```python
from build123d import *

# Parameters (mm, degrees)
SKETCH1_W              = 25.4
SKETCH1_H              = 25.4
SKETCH1_W_2            = 19.05
SKETCH1_H_2            = 19.05
EXTRUDE_THIN1_DEPTH    = 101.6
SKETCH2_R              = 9.525
CUT_EXTRUDE1_DEPTH     = 108.763073453
F_10_CLEARANCE_HOLE1_D = 5.1054


with BuildPart() as part:
    # Sketch1 → Extrude-Thin1 (new body)
    with BuildSketch(Plane.XY):
        with Locations((-12.7, 12.7)):
            Rectangle(SKETCH1_W, SKETCH1_H)
        with Locations((-12.7, 12.7)):
            Rectangle(SKETCH1_W_2, SKETCH1_H_2, mode=Mode.SUBTRACT)
    extrude(amount=EXTRUDE_THIN1_DEPTH)

    # Sketch2 → Cut-Extrude1 (cut, through all)
    with BuildSketch(Plane(origin=(0, 0, 0), x_dir=(-1, 0, 0), z_dir=(0, -1, 0))):
        with Locations(Location((12.7, -12.7, 0), (0, 0, 90))):
            Circle(SKETCH2_R)
    extrude(amount=-CUT_EXTRUDE1_DEPTH, mode=Mode.SUBTRACT)

    # #10 Clearance Hole1 (through all)
    with Locations(Plane(origin=(0, 0, 0), x_dir=(0, 0, -1), z_dir=(1, 0, 0))):
        with Locations((-76.2, 12.7), (-88.9, 12.7), (-63.5, 12.7)):
            Hole(F_10_CLEARANCE_HOLE1_D / 2)


solid = part.part
```
Could you check a few things on this model? Use its own coordinates, in mm. A direction names the side the tool comes from. Round coordinates to 2 decimals unless told otherwise and drop trailing zeros. Write each loop counter-clockwise with the first axis right and the second up, starting at its lowest first coordinate (ties: lowest second). Pieces come first, ordered by that corner, then holes. Notation, with made-up numbers: M -8.5,52 L 29.5,52 A21 ccw 29.5,73 Z; hole C -4,48 d3. An arc over 180 degrees is marked long. Write each question's results on one line, items separated by ' | '. Start each with the question number.
1. Imagine slicing it at C-C on z = 63.5. List the corners of the cut face in (x, y) for me (3 decimals).
2. On a 3-axis mill with a long thin cutter (end or side, diameter ignored), from which of +Z, -Z, +X, -X, +Y, -Y can I reach the whole of each face in a straight line? I mean faces 1 (the face through (-3.175, 13, 50)), 2 (the face through (-12.281, 23.79, 22.216)). Say none if no direction works.
3. I need wall thicknesses on L1, parallel to X at y = 21.75, z = 91 (3 decimals); L2, parallel to Y at x = -8, z = 65 (3 decimals); L3, parallel to Y at x = -2, z = 63.5. Which ranges of each line are inside material? Lowest first, please. Write a range as from..to.
4. Imagine slicing it at B-B on y = 7. List the corners of the cut face in (x, z) for me (3 decimals), and give its area (3 significant figures).
5. Imagine slicing it at D-D on y = 12.7. Count the separate pieces of the cut face and the enclosed holes in it, and give its area (3 significant figures).
6. Imagine slicing it at A-A on x = -23.5. List the corners of the cut face in (y, z) for me, and give its area (3 significant figures).
7. Thinking about a two-plate mould opening in X: for faces 3 (the face through (-13, 0, 61)), 4 (the face through (0, 13, 50)), 5 (the face through (-13, 22.225, 57)), which applies, +X half, -X half, draft (parallel to the pull), parting line (faces both ways), or undercut?
Result sheet:
1) outline: M -25.4,0 L 0,0 L 0,10.147 L -3.175,10.147 L -3.175,3.175 L -22.225,3.175 L -22.225,10.147 L -25.4,10.147 Z; M -25.4,15.253 L -22.225,15.253 L -22.225,22.225 L -3.175,22.225 L -3.175,15.253 L 0,15.253 L 0,25.4 L -25.4,25.4 Z
2) face 1: +Z, -Z | face 2: +Y, -Y
3) L1: x = -25.4..-22.225, -3.175..0 | L2: y = 0..3.175, 22.225..25.4 | L3: y = 0..10.15, 15.25..25.4
4) outline: M -25.4,0 L -22.225,0 L -22.225,101.6 L -25.4,101.6 Z; M -3.175,0 L 0,0 L 0,101.6 L -3.175,101.6 Z | area: 645 mm^2
5) separate pieces: 8 | enclosed holes: 0 | area: 548 mm^2
6) outline: M 0,0 L 25.4,0 L 25.4,101.6 L 0,101.6 Z; hole C 12.7,63.5 d5.11; hole C 12.7,76.2 d5.11; hole C 12.7,88.9 d5.11 | area: 2,520 mm^2
7) face 3: draft | face 4: +X half | face 5: undercut
